Geometry check sheet. Reference: the model listing, model coordinates, mm. A direction names the side the tool comes from. Coordinates: 2 decimals unless noted, no trailing zeros. Order: outer loops, then holes, each group sorted by start corner. A loop starts at its lowest first (then second) coordinate and runs counter-clockwise, first axis right, second up. Notation, with made-up numbers: (54, -38.5) -> (85, -38.5) arc R27 ccw to (85, -18.5) -> close; hole circle Ø10 at (51.25, -15). An arc over 180 degrees is marked (long way). Answer in a Markdown table with one row per item. Add a question column.
```python
from build123d import *

# Parameters (mm, degrees)
BOSS_EXTRUDE1_DEPTH = 6
FILLET1_R           = 3
SKETCH2_R           = 1.7
CUT_EXTRUDE1_DEPTH  = 42.743981602
FILLET2_SIZE        = 8
FILLET2_SIZE_2      = 2
FILLET3_SIZE        = 2
FILLET3_SIZE_2      = 10


# Some blends are built 0.0001 mm under size
with BuildPart() as part:
    # Sketch1 → Boss-Extrude1 (new body)
    with BuildSketch(Plane(origin=(0, 0, 0), x_dir=(1, 0, 0), z_dir=(0, 1, 0))):
        Polygon((0, 0), (0, 30), (5, 30), (5, 20), (23.4, 20), (23.4, 30), (28.4, 30), (28.4, 0), (23.4, 0), (23.4, 10), (5, 10), (5, 0), align=None)
    extrude(amount=BOSS_EXTRUDE1_DEPTH)

    # Fillet1
    fillet1_edges = [part.edges().sort_by_distance(p)[0] for p in [
        (2.5, 0, -30),
        (2.5, 6, -30),
        (25.9, 0, -30),
        (25.9, 6, -30),
        (2.5, 0, 0),
        (2.5, 6, 0),
        (25.9, 0, 0),
        (25.9, 6, 0),
    ]]
    fillet(fillet1_edges, radius=FILLET1_R - 0.0001)  # a hair under: the kernel refuses the full size

    # Sketch2 → Cut-Extrude1 (cut, through all)
    with BuildSketch(Plane(origin=(28.4, 0, 0), x_dir=(0, 0, -1), z_dir=(1, 0, 0))):
        with Locations((3, 3)):
            Circle(SKETCH2_R)
        with Locations((27, 3)):
            Circle(SKETCH2_R)
    extrude(amount=-CUT_EXTRUDE1_DEPTH, mode=Mode.SUBTRACT)

    # Fillet2
    # an asymmetric fillet: 8, 2 mm, written as the material it adds along each edge
    with BuildSketch(Plane(origin=(23.4, 0, -20), x_dir=(-1, 0, 0), z_dir=(0, 1, 0))) as fillet2_piece_1:
        with BuildLine():
            Bezier((FILLET2_SIZE, 0), (0, 0), (0, -FILLET2_SIZE_2), weights=[1, 0.707106781, 1])
            Line((0, -FILLET2_SIZE_2), (0, 0))
            Line((0, 0), (FILLET2_SIZE, 0))
        make_face()
    extrude(amount=6)
    with BuildSketch(Plane(origin=(5, 0, -10), x_dir=(0, 0, 1), z_dir=(0, 1, 0))) as fillet2_piece_2:
        with BuildLine():
            Bezier((FILLET2_SIZE_2, 0), (0, 0), (0, FILLET2_SIZE), weights=[1, 0.707106781, 1])
            Line((0, FILLET2_SIZE), (0, 0))
            Line((0, 0), (FILLET2_SIZE_2, 0))
        make_face()
    extrude(amount=6)

    # Fillet3
    # an asymmetric fillet: 10, 2 mm, written as the material it adds along each edge
    with BuildSketch(Plane(origin=(5, 0, -20), x_dir=(0, 0, -1), z_dir=(0, 1, 0))) as fillet3_piece_1:
        with BuildLine():
            Bezier((FILLET3_SIZE, 0), (0, 0), (0, -FILLET3_SIZE_2), weights=[1, 0.707106781, 1])
            Line((0, -FILLET3_SIZE_2), (0, 0))
            Line((0, 0), (FILLET3_SIZE, 0))
        make_face()
    extrude(amount=6)
    with BuildSketch(Plane(origin=(23.4, 0, -10), x_dir=(-1, 0, 0), z_dir=(0, 1, 0))) as fillet3_piece_2:
        with BuildLine():
            Bezier((FILLET3_SIZE_2, 0), (0, 0), (0, FILLET3_SIZE), weights=[1, 0.707106781, 1])
            Line((0, FILLET3_SIZE), (0, 0))
            Line((0, 0), (FILLET3_SIZE_2, 0))
        make_face()
    extrude(amount=6)


solid = part.part
```
(1) Cross-section at A-A (z = -7.5). Enter the section's corners in (x, y), plus the area to 3 significant figures.
(2) Cross-section at B-B (x = 24.75). Give the number of separate pieces and of enclosed holes in the cut face, plus the area to 3 significant figures.
(3) Go/stop test with a flat-tipped pin: P1, Ø2, axis at x = 13, y = 5, coming from the -Z side. Record where the tip stops, or that it passes through.
(4) Scan lines: line 1 along Y through (x, z) = (25.3, -27); line 2 along X through (y, z) = (5.5, -22.25); line 3 along Z through (x, y) = (13.75, 2). Record each from-to range of solid material in increasing order.
(5) Mould release check, pull along Y, two halves, no side actions. Record for faces 1 (the face through (25.94, 0.9, -29.14)), 2 (the face through (23.4, 3, -25)), 3 (the face through (2.54, 3.51, -4.62)): +Y half, -Y half, draft (parallel to the pull), parting line (faces both ways), or undercut.
(6) Access from +Z, -Z, +X, -X, +Y, -Y to the whole of each face (thin tool, end or side, straight path). Record for faces 4 (the face through (25.94, 2.35, -28.57)), 5 (the face through (5, 3, -25)), 6 (the face through (23.4, 3, -5)).
Checks:
| question | item | result |
|---|---|---|
| 1 | outline | (0, 0) -> (5, 0) -> (5, 6) -> (0, 6) -> close; (23.4, 0) -> (28.4, 0) -> (28.4, 6) -> (23.4, 6) -> close |
| 1 | area | 60.0 mm² |
| 2 | separate pieces | 1 |
| 2 | enclosed holes | 2 |
| 2 | area | 154 mm² |
| 3 | P1 | z = -20.09 |
| 4 | line 1 | 0 to 1.3, 4.7 to 6 |
| 4 | line 2 | 0 to 5, 23.4 to 28.4 |
| 4 | line 3 | -20.02 to -10 |
| 5 | face 1 | -Y half |
| 5 | face 2 | draft |
| 5 | face 3 | undercut |
| 6 | face 4 | +X, -X |
| 6 | face 5 | -Z, +Y, -Y |
| 6 | face 6 | +Z, +Y, -Y |
